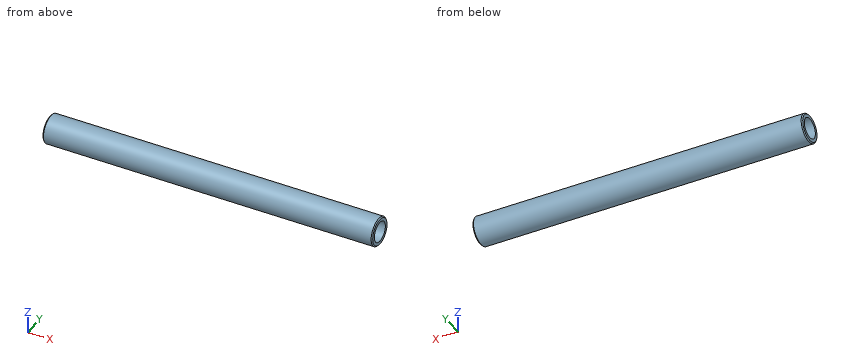
```python
from build123d import *

# Parameters (mm, degrees)
F0_W    = 133.35
F0_H    = 3.175
F0_W_2  = 12.7
F0_W_3  = 114.3
F2_SIZE = 0.8128
F3_SIZE = 0.8128


with BuildPart() as f1:
    # F0 (on Front) → F1 (revolve)
    with BuildSketch(Plane.XZ):
        with Locations((-71.7826074213, 0.0330159035)):
            Rectangle(F0_W, F0_H)
        with Locations((115.5423925787, 0.0330159035)):
            Rectangle(F0_W_2, F0_H)
        with Locations((52.0423925787, 0.0330159035)):
            Rectangle(F0_W_3, F0_H)
    revolve(axis=Axis((-8.2826074213, 0, -9.4792840965), (1, 0, 0)))

    # F2
    f2_edges = [f1.edges().sort_by_distance(p)[0] for p in [
        (121.892393, 0, -20.579084),
    ]]
    chamfer(f2_edges, length=F2_SIZE)

    # F3
    f3_edges = [f1.edges().sort_by_distance(p)[0] for p in [
        (-138.457607, 0, -20.579084),
    ]]
    chamfer(f3_edges, length=F3_SIZE)


solid = f1.part
```
Can you work these out from the model? Positions are in its coordinate system, mm. Coordinates: 2 decimals unless noted, no trailing zeros. Loops run counter-clockwise (first coordinate to the right, second up) from the corner with the lowest first, then second, coordinate; pieces in that order, holes last. Notation, with made-up numbers: M 71,71 L 110,71 A17 cw 110,98 Z; hole C 88,-15 d2. An arc over 180 degrees is marked long. Put each result on its own line as item: value. Start each with the question number.
(1) Will these pins go through, and if not, where does the flat tip stop? pin 1 Ø12.5 at (y, z) = (0, -9.48) entering from +X; pin 2 Ø1.5 at (x, y) = (-50, -2) entering from +Z; pin 3 Ø1.5 at (x, y) = (49.5, -3) entering from +Z.
(2) Imagine slicing it at B-B on x = -36.5. List the corners of the cut face in (y, z) for me.
(3) I need wall thicknesses on probe 1 along Y at (x, z) = (43.5, -10.25); probe 2 along Z at (x, y) = (-76, 0); probe 3 along Z at (x, y) = (50, 3.75). Which ranges of each line are inside material? Lowest first, please.
(4) Imagine slicing it at A-A on y = 0. List the corners of the cut face in (x, z) for me.
Worked answers:
1. pin 1: passes through
1. pin 2: stops at z = 1.55
1. pin 3: stops at z = 1.39
2. outline: C 0,-9.48 d22.2; hole C 0,-9.48 d15.85
3. probe 1: y = -11.07 to -7.89, 7.89 to 11.07
3. probe 2: z = -20.58 to -17.4, -1.55 to 1.62
3. probe 3: z = -19.93 to -16.46, -2.5 to 0.97
4. outline: M -138.46,-19.77 L -137.64,-20.58 L 121.08,-20.58 L 121.89,-19.77 L 121.89,-17.4 L -138.46,-17.4 Z; M -138.46,-1.55 L 121.89,-1.55 L 121.89,0.81 L 121.08,1.62 L -137.64,1.62 L -138.46,0.81 Z
